Part model, mm, in its own coordinate system. Face numbers are marked on the shaded views. Give positions to 0.01 mm unless a question says otherwise; leave off trailing zeros. Order: outer loops, then holes, each group sorted by start corner. A loop starts at its lowest first (then second) coordinate and runs counter-clockwise, first axis right, second up. Notation, with made-up numbers: (-3, 70.5) -> (34, 70.5) arc R34 ccw to (34, 103.5) -> close; hole circle Ø4 at (58.5, 6). An arc over 180 degrees is marked (long way). Write item = value, one per line. Start each with the question number.
Item 1: Band-saw the part on B-B on x = -14. Write the cut outline in (y, z).
Item 2: Band-saw the part on A-A on z = -2.5. Write the cut outline in (x, y).
Item 3: Band-saw the part on C-C on z = -8.75. Write the cut outline in (x, y).
Item 4: Pull direction Y, two halves, no side cores. Call the marked faces 1, 2, 3 and 4: +Y half, -Y half, draft (parallel to the pull), parting line (faces both ways), or undercut.
Item 5: Drill centre lines: line 1 along X through (y, z) = (-15.6, -14.5); line 2 along X through (y, z) = (-2, 1.5); line 3 along Y through (x, z) = (36, -5.5). Where is each one in solid material? Low to high.
Item 6: Flat gauge pins, fed straight in: P1, Ø12, axis at y = -6.5, z = -5.5, coming from the -X side; P2, Ø3.5, axis at x = 14.5, y = 2.5, coming from the -Z side; P3, Ø3.5, axis at x = -75.75, z = -8.63, coming from the +Y side. Where does each tip first touch, or does it go through?
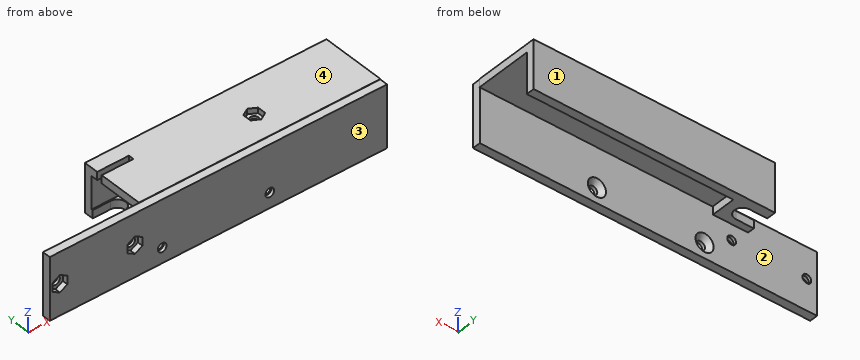
```python
from build123d import *

# Parameters (mm, degrees)
CROQUIS1_R                      = 1.625
SALIENTE_EXTRUIR1_DEPTH         = 3
CORTAR_EXTRUIR1_DEPTH           = 2
CROQUIS3_W                      = 125
CROQUIS3_H                      = 23
CROQUIS3_R                      = 1.625
SALIENTE_EXTRUIR2_DEPTH         = 3
CROQUIS4_W                      = 76
CROQUIS4_H                      = 15
SALIENTE_EXTRUIR3_DEPTH         = 3
SALIENTE_EXTRUIR5_DEPTH         = 13.5
CROQUIS18_W                     = 13
CROQUIS18_H                     = 12
SALIENTE_EXTRUIR6_DEPTH         = 3
CORTAR_EXTRUIR6_DEPTH           = 3
CROQUIS21_W                     = 76.5
CROQUIS21_H                     = 3
SALIENTE_EXTRUIR7_DEPTH         = 3
CROQUIS23_W                     = 11.762217651
CROQUIS23_H                     = 2
CORTAR_EXTRUIR7_DEPTH           = 3
CROQUIS24_R                     = 3.35997123
CORTAR_EXTRUIR8_DEPTH           = 1.8
CORTAR_EXTRUIR8_DRAFT           = -44
CORTAR_EXTRUIR8_PROFILE_2_DEPTH = 1.8
CORTAR_EXTRUIR8_PROFILE_2_DRAFT = -44
CORTAR_EXTRUIR9_DEPTH           = 2


with BuildPart() as part:
    # Croquis1 → Saliente-Extruir1 (new body)
    with BuildSketch(Plane.XY):
        Polygon((7.541029965, -13.191741873), (45.541029965, -13.191741873), (45.541029965, 7.808258127), (-30.458970035, 7.808258127), (-30.458970035, -13.191741873), align=None)
        with Locations((7.541029965, -2.691741873)):
            Circle(CROQUIS1_R, mode=Mode.SUBTRACT)
    extrude(amount=SALIENTE_EXTRUIR1_DEPTH)

    # Croquis2 → Cortar-Extruir1 (cut)
    with BuildSketch(Plane.XY.offset(3)):
        Polygon((7.541029965, 0.478258127), (4.795729435, -1.106741873), (4.795729435, -4.276741873), (7.541029965, -5.861741873), (10.286330495, -4.276741873), (10.286330495, -1.106741873), align=None)
    extrude(amount=-CORTAR_EXTRUIR1_DEPTH, mode=Mode.SUBTRACT)

    # Croquis3 → Saliente-Extruir2 (add)
    with BuildSketch(Plane.XZ.offset(13.191741873)):
        with Locations((-17.025379291, -8.632818511)):
            Rectangle(CROQUIS3_W, CROQUIS3_H)
        with Locations(Location((2.041029965, -14.5, 0), (0, 0, 270))):
            Circle(CROQUIS3_R, mode=Mode.SUBTRACT)
        with Locations(Location((-37.853447155, -14.5, 0), (0, 0, 270))):
            Circle(CROQUIS3_R, mode=Mode.SUBTRACT)
        with Locations(Location((-75.748970035, -8.632818511, 0), (0, 0, 270))):
            Circle(CROQUIS3_R, mode=Mode.SUBTRACT)
        with Locations(Location((-47.888970035, -8.632818511, 0), (0, 0, 270))):
            Circle(CROQUIS3_R, mode=Mode.SUBTRACT)
    extrude(amount=SALIENTE_EXTRUIR2_DEPTH)

    # Croquis4 → Saliente-Extruir3 (add)
    with BuildSketch(Plane(origin=(0, 7.808258127, 0), x_dir=(1, 0, 0), z_dir=(0, 1, 0))):
        with Locations((7.541029965, 4.5)):
            Rectangle(CROQUIS4_W, CROQUIS4_H)
    extrude(amount=SALIENTE_EXTRUIR3_DEPTH)

    # Croquis14 → Saliente-Extruir5 (add)
    with BuildSketch(Plane.ZY.offset(30.458970035)):
        Polygon((-12, 10.808258127), (3, 10.808258127), (3, -13.191741873), (0, -13.191741873), (0, 7.808258127), (-12, 7.808258127), align=None)
    extrude(amount=SALIENTE_EXTRUIR5_DEPTH)

    # Croquis18 → Saliente-Extruir6 (add)
    with BuildSketch(Plane(origin=(0, 0, -12), x_dir=(-1, 0, 0), z_dir=(0, 0, -1))):
        with Locations((37.458970035, 4.808258127)):
            Rectangle(CROQUIS18_W, CROQUIS18_H)
    extrude(amount=SALIENTE_EXTRUIR6_DEPTH)

    # Croquis19 → Cortar-Extruir6 (cut)
    with BuildSketch(Plane(origin=(0, 0, -15), x_dir=(-1, 0, 0), z_dir=(0, 0, -1))):
        with BuildLine():
            Line((37.340127553, 7.35825754), (43.958970035, 7.35825754))
            Line((43.958970035, 7.35825754), (43.958970035, 1.358257834))
            Line((43.958970035, 1.358257834), (37.340127553, 1.358257834))
            ThreePointArc((37.340127553, 1.358257834), (34.310076321, 4.358257687), (37.340127553, 7.35825754))
        make_face()
    extrude(amount=-CORTAR_EXTRUIR6_DEPTH, mode=Mode.SUBTRACT)

    # Croquis21 → Saliente-Extruir7 (add)
    with BuildSketch(Plane(origin=(0, 10.808258127, 0), x_dir=(1, 0, 0), z_dir=(0, 1, 0))):
        with Locations((7.291029965, 13.5)):
            Rectangle(CROQUIS21_W, CROQUIS21_H)
    extrude(amount=-SALIENTE_EXTRUIR7_DEPTH)

    # Croquis23 → Cortar-Extruir7 (cut)
    with BuildSketch(Plane.XY.offset(3)):
        with Locations((-38.077861209, 4.358257834)):
            Rectangle(CROQUIS23_W, CROQUIS23_H)
    extrude(amount=-CORTAR_EXTRUIR7_DEPTH, mode=Mode.SUBTRACT)


with BuildPart() as cortar_extruir8_tool:
    # Croquis24 → Cortar-Extruir8 (with draft: the straight prism first)
    with BuildSketch(Plane(origin=(0, -13.191741873, 0), x_dir=(1, 0, 0), z_dir=(0, 1, 0))):
        with Locations((2.041029965, 14.5)):
            Circle(CROQUIS24_R)
    extrude(amount=-CORTAR_EXTRUIR8_DEPTH)
    # Cortar-Extruir8: the draft: its side faces are tilted about the plane it starts from
    cortar_extruir8_sides = [cortar_extruir8_tool.faces().sort_by_distance(p)[0] for p in [
        (-1.318941265, -14.091741873, -14.5),
    ]]
    draft(cortar_extruir8_sides, Plane(origin=(0, -13.191741873, 0), x_dir=(1, 0, 0), z_dir=(0, 1, 0)), CORTAR_EXTRUIR8_DRAFT)


with BuildPart() as part_1:
    add(part.part)

    # Cortar-Extruir8: cut by cortar_extruir8_tool
    add(cortar_extruir8_tool.part, mode=Mode.SUBTRACT)


with BuildPart() as cortar_extruir8_profile_2_tool:
    # Croquis24 → Cortar-Extruir8 profile 2 (with draft: the straight prism first)
    with BuildSketch(Plane(origin=(0, -13.191741873, 0), x_dir=(1, 0, 0), z_dir=(0, 1, 0))):
        with Locations((-37.853447155, 14.5)):
            Circle(CROQUIS24_R)
    extrude(amount=-CORTAR_EXTRUIR8_PROFILE_2_DEPTH)
    # Cortar-Extruir8 profile 2: the draft: its side faces are tilted about the plane it starts from
    cortar_extruir8_profile_2_sides = [cortar_extruir8_profile_2_tool.faces().sort_by_distance(p)[0] for p in [
        (-41.213418385, -14.091741873, -14.5),
    ]]
    draft(cortar_extruir8_profile_2_sides, Plane(origin=(0, -13.191741873, 0), x_dir=(1, 0, 0), z_dir=(0, 1, 0)), CORTAR_EXTRUIR8_PROFILE_2_DRAFT)


with BuildPart() as part_2:
    add(part_1.part)

    # Cortar-Extruir8 profile 2: cut by cortar_extruir8_profile_2_tool
    add(cortar_extruir8_profile_2_tool.part, mode=Mode.SUBTRACT)

    # Croquis25 → Cortar-Extruir9 (cut)
    with BuildSketch(Plane.XZ.offset(16.191741873)):
        Polygon((-47.922954999, -5.403954828), (-50.668255529, -6.988954828), (-50.668255529, -10.158954828), (-47.922954999, -11.743954828), (-45.177654469, -10.158954828), (-45.177654469, -6.988954828), align=None)
        Polygon((-75.748970035, -5.462818511), (-78.494270565, -7.047818511), (-78.494270565, -10.217818511), (-75.748970035, -11.802818511), (-73.003669505, -10.217818511), (-73.003669505, -7.047818511), align=None)
    extrude(amount=-CORTAR_EXTRUIR9_DEPTH, mode=Mode.SUBTRACT)


solid = part_2.part
```
Values found:
q1.outline = (-16.19, -20.13) -> (-13.19, -20.13) -> (-13.19, 0) -> (7.81, 0) -> (7.81, -15) -> (10.81, -15) -> (10.81, 3) -> (-13.19, 3) -> (-13.19, 2.87) -> (-16.19, 2.87) -> close
q2.outline = (-79.53, -16.19) -> (45.47, -16.19) -> (45.47, -13.19) -> (-79.53, -13.19) -> close; (-43.96, 7.81) -> (45.54, 7.81) -> (45.54, 10.81) -> (-43.96, 10.81) -> close
q3.outline = (-79.53, -16.19) -> (-78.49, -16.19) -> (-78.49, -14.19) -> (-77.37, -14.19) -> (-77.37, -13.19) -> (-79.53, -13.19) -> close; (-74.13, -14.19) -> (-73, -14.19) -> (-73, -16.19) -> (-50.67, -16.19) -> (-50.67, -14.19) -> (-49.51, -14.19) -> (-49.51, -13.19) -> (-74.13, -13.19) -> close; (-46.27, -14.19) -> (-45.18, -14.19) -> (-45.18, -16.19) -> (45.47, -16.19) -> (45.47, -13.19) -> (-46.27, -13.19) -> close; (-43.96, 7.81) -> (45.54, 7.81) -> (45.54, 10.81) -> (-43.96, 10.81) -> close
q4.face_1 = +Y half
q4.face_2 = undercut
q4.face_3 = -Y half
q4.face_4 = draft
q5.line_1 = -79.53 to -39.48, -36.23 to 0.42, 3.67 to 45.47
q5.line_2 = -43.96 to 4.8, 10.29 to 45.54
q5.line_3 = -16.19 to -13.19, 7.81 to 10.81
q6.P1 = -43.96
q6.P2 = 0
q6.P3 = -13.19
